Study the drawing (mm; zero at the part's minimum x, y, z) and answer. A direction names the side the tool comes from. Coordinates: 2 decimals unless noted, no trailing zeros. Loops run counter-clockwise (first coordinate to the right, second up) from the corner with the lowest first, then second, coordinate; pieces in that order, holes last. Notation, with made-up numbers: (19, 76) - (45, 76) arc R18 ccw to (45, 101) - close; hole circle Ø3 at (42, 81.25). An arc over 180 degrees is marked (long way). Use CSV: the item, a comma, the result in double quotes.
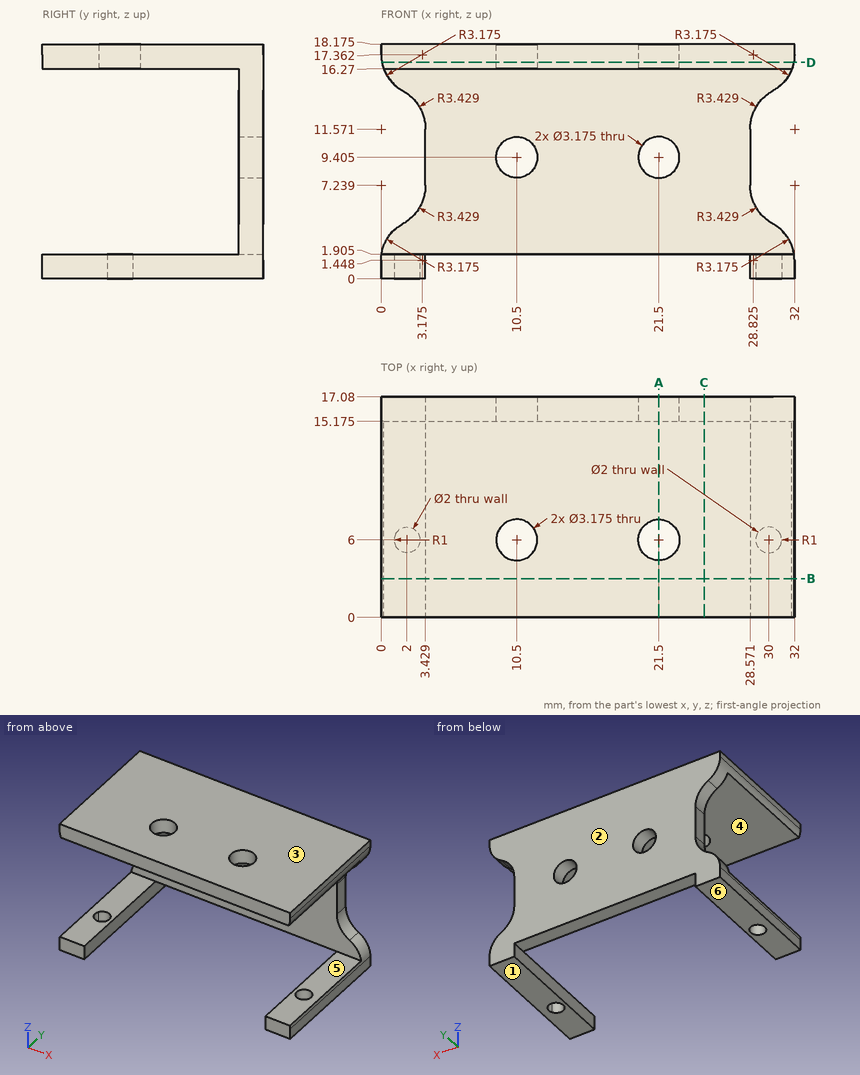
Q1. The part is cut by section C-C on x = 25. Determine the outline of the cut face in (y, z) (1 decimal).
Reported:
outline,"(0, 16.3) - (15.2, 16.3) - (15.2, 1.9) - (17.1, 1.9) - (17.1, 18.2) - (0, 18.2) - close"
Q2. Given P1, Ø1, axis at x = 6, z = 12, coming from the -Y side (3 decimals); P2, Ø2.5, axis at x = 10.5, z = 9.405, coming from the -Y side; P3, Ø1.2, axis at x = 2, y = 6, coming from the -Z side; P4, Ø10, axis at y = 12.5, z = 11.5, coming from the +X side, each flat-ended and moving along its own axis, determine where each tip first touches the part or whether it passes through.
Reported:
P1,"stops at y = 15.175"
P2,"passes through"
P3,"stops at z = 16.27"
P4,"stops at x = 31.88"
Q3. For a pull along Z with two mould halves and no side action, classify the marked faces 1, 2, 3 and 4 as +Z half, -Z half, draft (parallel to the pull), parting line (faces both ways), or undercut.
Reported:
face 1,"-Z half"
face 2,"draft"
face 3,"+Z half"
face 4,"undercut"
Q4. A tool of negligible diameter and unlimited length cuts with its end or side. For the marked faces 5 and 6, from which of +Z, -Z, +X, -X, +Y, -Y can it reach the whole face along a straight path? Write none if from no direction.
Reported:
face 5,"+X, -X, -Y"
face 6,"-Z, +X, -X, +Y, -Y"
Q5. The part is cut by section D-D on z = 16.75. Determine the outline of the cut face in (x, y) (1 decimal), and give its area (3 significant figures).
Reported:
outline,"(0.1, 0) - (31.9, 0) - (31.9, 17.1) - (0.1, 17.1) - close; hole circle Ø3.2 at (10.5, 6); hole circle Ø3.2 at (21.5, 6)"
area,"529 mm²"
Q6. The part is cut by section A-A on x = 21.5. Determine the outline of the cut face in (y, z) (1 decimal), and give its area (3 significant figures).
Reported:
outline,"(0, 16.3) - (4.4, 16.3) - (4.4, 18.2) - (0, 18.2) - close; (7.6, 16.3) - (15.2, 16.3) - (15.2, 11) - (17.1, 11) - (17.1, 18.2) - (7.6, 18.2) - close; (15.2, 1.9) - (17.1, 1.9) - (17.1, 7.8) - (15.2, 7.8) - close"
area,"47.8 mm²"
Q7. Find the intervals of material crossed by probe 1 along X at (y, z) = (6, 0.4); probe 2 along Z at (x, y) = (21.5, 15.9) (1 decimal); probe 3 along X at (y, z) = (12.75, 1), in increasing order. Write a range as [from, to].
Reported:
probe 1,"x = [0, 1], [3, 3.43], [28.57, 29], [31, 32]"
probe 2,"z = [1.9, 7.8], [11, 18.2]"
probe 3,"x = [0, 3.43], [28.57, 32]"
Q8. The part is cut by section B-B on y = 3. Give the number of separate pieces and of enclosed holes in the cut face.
Reported:
separate pieces,"3"
enclosed holes,"0"
